Can you work these out from the drawing? Everything is in mm from the part's minimum corner. Coordinates: 2 decimals unless noted, no trailing zeros. Loops run counter-clockwise (first coordinate to the right, second up) from the corner with the lowest first, then second, coordinate; pieces in that order, holes last.
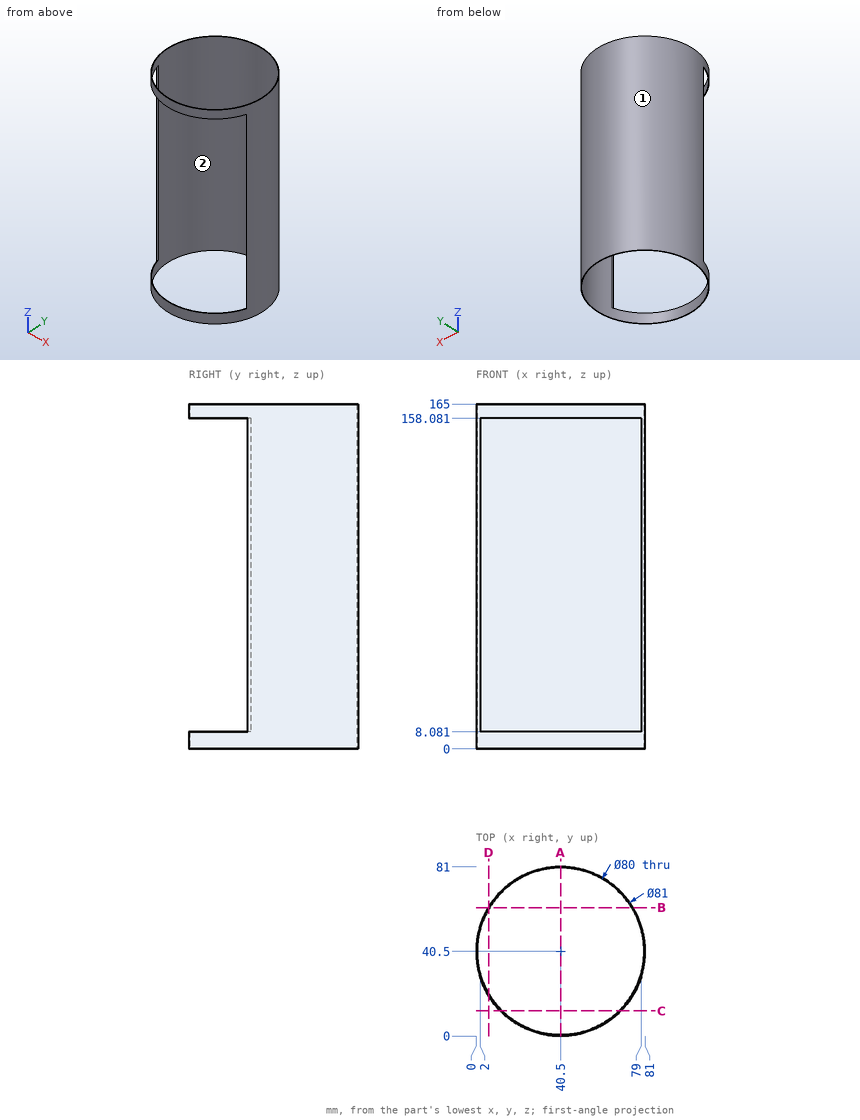
(1) Imagine slicing it at D-D, the plane x = 6. Write out the boundary of the cut face in (y, z), and give its area (3 significant figures).
Answers:
outline: (19.29, 0) - (20.26, 0) - (20.26, 8.08) - (19.29, 8.08) - close; (19.29, 158.08) - (20.26, 158.08) - (20.26, 165) - (19.29, 165) - close; (60.74, 0) - (61.71, 0) - (61.71, 165) - (60.74, 165) - close
area: 175 mm2
(2) We'd pull the mould along X, two halves only. Please class the marked faces 1 and 2: +X half, -X half, draft (parallel to the pull), parting line (faces both ways), or undercut.
Answers:
face 1: parting line
face 2: undercut
(3) Imagine slicing it at A-A, the plane x = 40.5. Write out the boundary of the cut face in (y, z).
Answers:
outline: (0, 0) - (0.5, 0) - (0.5, 8.08) - (0, 8.08) - close; (0, 158.08) - (0.5, 158.08) - (0.5, 165) - (0, 165) - close; (80.5, 0) - (81, 0) - (81, 165) - (80.5, 165) - close
(4) Imagine slicing it at B-B, the plane y = 61.5. Write out the boundary of the cut face in (x, z).
Answers:
outline: (5.87, 0) - (6.46, 0) - (6.46, 165) - (5.87, 165) - close; (74.54, 0) - (75.13, 0) - (75.13, 165) - (74.54, 165) - close
(5) I need wall thicknesses on probe 1 along X at (y, z) = (42, 84.5); probe 2 along Y at (x, z) = (40.5, 61.5); probe 3 along X at (y, z) = (28.5, 144.5). Which ranges of each line are inside material? Lowest first, please.
Answers:
probe 1: x = 0.03 to 0.53, 80.47 to 80.97
probe 2: y = 80.5 to 81
probe 3: x = 1.82 to 2, 79 to 79.18
(6) Imagine slicing it at C-C, the plane y = 12. Write out the boundary of the cut face in (x, z) (3 decimals).
Answers:
outline: (11.725, 0) - (12.433, 0) - (12.433, 8.081) - (11.725, 8.081) - close; (11.725, 158.081) - (12.433, 158.081) - (12.433, 165) - (11.725, 165) - close; (68.567, 0) - (69.275, 0) - (69.275, 8.081) - (68.567, 8.081) - close; (68.567, 158.081) - (69.275, 158.081) - (69.275, 165) - (68.567, 165) - close
(7) For pin 1 (6 mm diameter, centred on x = 63.5, z = 20.5, fed in from -Y); pin 2 (3 mm diameter, centred on x = 22.5, z = 58.5, fed in from -Y) (3 decimals); pin 3 (1.5 mm diameter, centred on y = 61.5, z = 94, fed in from +X), each with a flat end and sliding along its axis, tell me the tip position at first contact or that it passes through.
Answers:
pin 1: stops at y = 70.9
pin 2: stops at y = 75.425
pin 3: stops at x = 75.57
